Work out the finished part from the listing and answer in its coordinate system (mm). A direction names the side the tool comes from. Give positions to 0.01 mm unless a question says otherwise; leave off trailing zeros. Loops run counter-clockwise (first coordinate to the right, second up) from the corner with the lowest first, then second, coordinate; pieces in that order, holes last. Notation, with made-up numbers: (35, 36.25) - (59, 36.25) arc R26 cw to (59, 75.25) - close; hole circle Ø4 at (22, 68.25). An arc over 180 degrees is marked (long way). One line per item, written item: value.
from build123d import *

# Parameters (mm, degrees)
PAD017_DEPTH           = 5
PAD020_DEPTH           = 6.25
SKETCH038_W            = 10
SKETCH038_H            = 1.65
PAD021_DEPTH           = 5
SKETCH079_W            = 15.2
SKETCH079_H            = 1.65
PAD051_DEPTH           = 2.1
SKETCH080_W            = 7.1
SKETCH080_H            = 1.65
PAD052_DEPTH           = 5
SKETCH081_W            = 15.2
SKETCH081_H            = 1.65
PAD053_DEPTH           = 5
LINEARPATTERN018_COUNT = 2
LINEARPATTERN018_PITCH = 3.3
CHAMFER008_SIZE        = 1


with BuildPart() as obj1:
    # Sketch034 → Pad017 (new body)
    with BuildSketch(Plane.XY):
        with BuildLine():
            Line((-1.35, -1.8), (-1.35, 6))
            ThreePointArc((0, 7.35), (-0.954594, 6.954594), (-1.35, 6))
            Line((0, 9), (0, 7.35))
            Line((-2.6, 9), (0, 9))
            Line((-2.6, -1.8), (-2.6, 9))
            Line((-3.85, -1.8), (-2.6, -1.8))
            ThreePointArc((-3.85, -1.8), (-3.439949, -2.789949), (-2.45, -3.2))
            Line((-1.35, -3.2), (-2.45, -3.2))
            Line((-1.35, -1.8), (-1.35, -3.2))
        make_face()
    extrude(amount=PAD017_DEPTH)

    # Sketch037 → Pad020 (join)
    with BuildSketch(Plane.XY):
        Polygon((-1.35, 0.2), (-1.35, 1.6), (-2.6, 1.6), (-3.85, 1.6), (-3, 0.2), (-2.6, 0.2), align=None)
    extrude(amount=PAD020_DEPTH)


with BuildPart() as body028:
    # Mirror002: instance of _obj1
    add(obj1.part.mirror(Plane(origin=(5, 0, 0), x_dir=(0, 1, 0), z_dir=(-1, 0, 0))))

    # Fusion002: union _obj1
    add(obj1.part)


with BuildPart() as body028_1:
    # Clone003 placement: moved
    add(body028.part.moved(Location((-5, 0, 0))))

    # Sketch038 → Pad021 (new body)
    with BuildSketch(Plane.XY):
        with Locations((0, 8.175)):
            Rectangle(SKETCH038_W, SKETCH038_H)
    extrude(amount=PAD021_DEPTH)

    # Sketch079 → Pad051 (new body)
    with BuildSketch(Plane.XY):
        with Locations((0, 9.825)):
            Rectangle(SKETCH079_W, SKETCH079_H)
    pad051 = extrude(amount=PAD051_DEPTH)

    # Sketch080 → Pad052 (join)
    with BuildSketch(Plane.XY):
        with Locations((4.05, 9.825)):
            Rectangle(SKETCH080_W, SKETCH080_H)
    pad052 = extrude(amount=PAD052_DEPTH)

    # Sketch081 → Pad053 (join)
    with BuildSketch(Plane.XY):
        with Locations((0, 11.475)):
            Rectangle(SKETCH081_W, SKETCH081_H)
    pad053 = extrude(amount=PAD053_DEPTH)

    # LinearPattern018: Pad053, Pad052, Pad051 ×2
    with Locations(*[(0, i * LINEARPATTERN018_PITCH, 0) for i in range(1, LINEARPATTERN018_COUNT)]):
        add(pad053)
        add(pad052)
        add(pad051)

    # Chamfer008
    chamfer008_edges = [body028_1.edges().sort_by_distance(p)[0] for p in [
        (-7.6, 5.3, 5),
        (-7.6, 11.475, 5),
        (-7.6, 14.775, 5),
    ]]
    chamfer(chamfer008_edges, length=CHAMFER008_SIZE)


with BuildPart() as body028_2:
    # Body028 placement: moved
    add(body028_1.part.moved(Location((-5, 0, 0))))


solid = body028_2.part
1. For faces 1 (the flat face through (-13.43, 0.91, 3.08)), 2 (the flat face through (-12.1, 5.2, 4.5)), 3 (the flat face through (-12, -2, 5)), determine the directions among +Z, -Z, +X, -X, +Y, -Y from which every point of the face is accessible in a straight line to the end or side of a thin tool.
Output:
face 1: +Z, -Z, -X
face 2: +Z, -X, +Y
face 3: +Z, +X, -X, -Y
2. Flat-ended cylindrical pins translate along their axes: pin 1 Ø3 at (x, y) = (-12.5, -2) entering from +Z; pin 2 Ø1 at (x, y) = (-10.5, 8.5) entering from -Z; pin 3 Ø3 at (x, z) = (-7.5, 3.5) entering from -Y; pin 4 Ø0.8 at (x, y) = (-8.5, 13) entering from +Z. Find the tip coordinate at first contact, or state that the pin passes through.
Output:
pin 1: stops at z = 5
pin 2: stops at z = 0
pin 3: stops at y = 7.35
pin 4: stops at z = 2.1
3. Section C-C (z = 5.5) is taken. Write down the section's boundary in (x, y), and give its area (3 significant figures).
Output:
outline: (-13.85, 1.6) - (-13, 0.2) - (-11.35, 0.2) - (-11.35, 1.6) - close; (1.35, 0.2) - (3, 0.2) - (3.85, 1.6) - (1.35, 1.6) - close
area: 5.81 mm²
4. Section B-B (x = -8.25) is taken. Write down the section's boundary in (y, z), and give its area (3 significant figures).
Output:
outline: (7.35, 0) - (15.6, 0) - (15.6, 5) - (13.95, 5) - (13.95, 2.1) - (12.3, 2.1) - (12.3, 5) - (10.65, 5) - (10.65, 2.1) - (9, 2.1) - (9, 5) - (7.35, 5) - close
area: 31.7 mm²
5. Find the intervals of material crossed by line 1 along Y through (x, z) = (-5.75, 4.5); line 2 along X through (y, z) = (5.75, 3.5); line 3 along X through (y, z) = (11.25, 3.75), in increasing order.
Output:
line 1: y = 7.35 to 9, 10.65 to 12.3, 13.95 to 15.6
line 2: x = -12.6 to -11.35, 1.35 to 2.6
line 3: x = -12.6 to 2.6
6. The mould has two halves that part along X. Classify faces 4 (the flat face through (2.6, 0.2, 5.2)), 5 (the cylindrical face through (-13.45, -2.78, 2.46)), 6 (the flat face through (1.35, 1, 2)): released by +X, released by -X, zero draft, split by the parting line, or undercut.
Output:
face 4: zero draft
face 5: released by -X
face 6: undercut
7. Section A-A (y = -1) is taken. Write down the section's boundary in (x, z).
Output:
outline: (-12.6, 0) - (-11.35, 0) - (-11.35, 5) - (-12.6, 5) - close; (1.35, 0) - (2.6, 0) - (2.6, 5) - (1.35, 5) - close
